Check sheet for the drawn part. Datum: minimum x, y, z corner. Units: mm. Round coordinates to 2 decimals unless told otherwise and drop trailing zeros. Write each loop counter-clockwise with the first axis right and the second up, starting at its lowest first coordinate (ties: lowest second). Pieces come first, ordered by that corner, then holes. Notation, with made-up numbers: (87, -20.75) - (142, -20.75) arc R22 cw to (142, 13.25) - close; hole circle Ø4 at (-20, 5.5). An arc over 180 degrees is marked (long way). Answer as a JSON object with one key per item and string values.
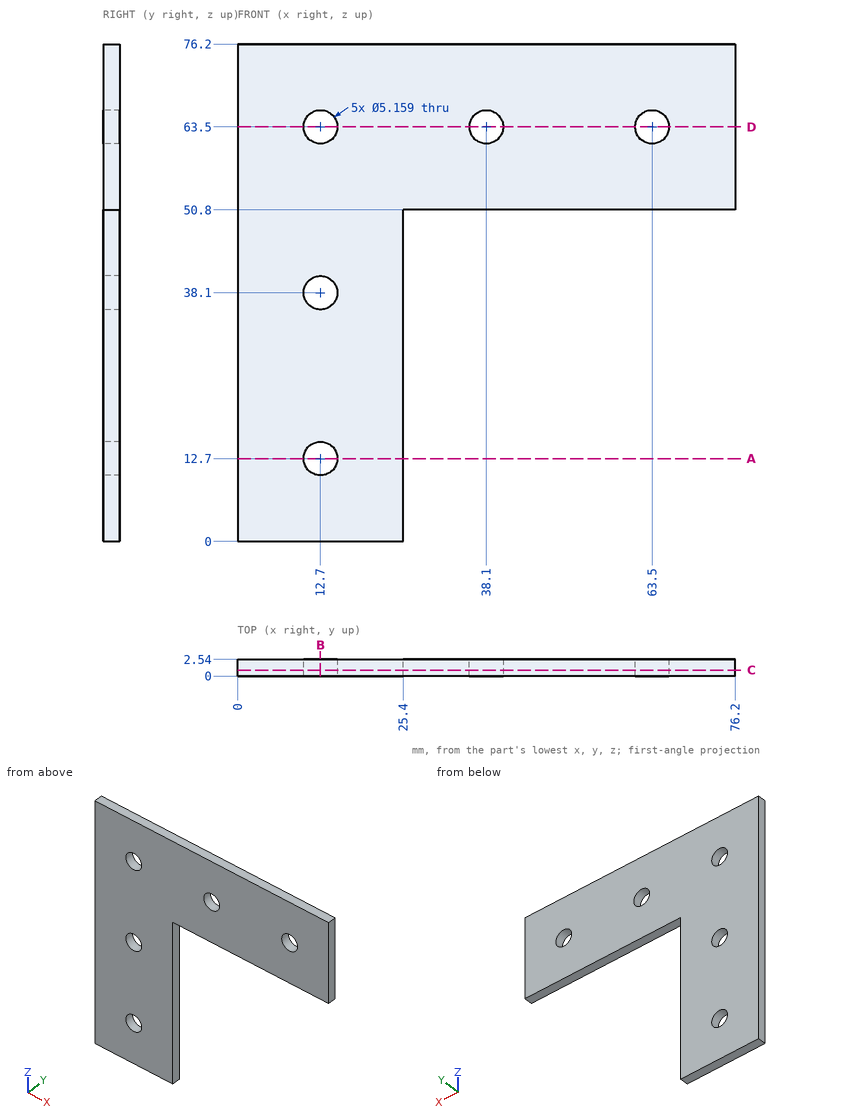
1. Cross-section at D-D (z = 63.5). Record the boundary of the cut face in (x, y).
Completed:
{"outline": "(0, 0) - (10.12, 0) - (10.12, 2.54) - (0, 2.54) - close; (15.28, 0) - (35.52, 0) - (35.52, 2.54) - (15.28, 2.54) - close; (40.68, 0) - (60.92, 0) - (60.92, 2.54) - (40.68, 2.54) - close; (66.08, 0) - (76.2, 0) - (76.2, 2.54) - (66.08, 2.54) - close"}
2. Cross-section at C-C (y = 0.9). Record the boundary of the cut face in (x, z), plus the area to 3 significant figures.
Completed:
{"outline": "(0, 0) - (25.4, 0) - (25.4, 50.8) - (76.2, 50.8) - (76.2, 76.2) - (0, 76.2) - close; hole circle Ø5.16 at (12.7, 12.7); hole circle Ø5.16 at (12.7, 38.1); hole circle Ø5.16 at (12.7, 63.5); hole circle Ø5.16 at (38.1, 63.5); hole circle Ø5.16 at (63.5, 63.5)", "area": "3,120 mm^2"}
3. Cross-section at B-B (x = 12.7). Record the boundary of the cut face in (y, z), plus the area to 3 significant figures.
Completed:
{"outline": "(0, 0) - (2.54, 0) - (2.54, 10.12) - (0, 10.12) - close; (0, 15.28) - (2.54, 15.28) - (2.54, 35.52) - (0, 35.52) - close; (0, 40.68) - (2.54, 40.68) - (2.54, 60.92) - (0, 60.92) - close; (0, 66.08) - (2.54, 66.08) - (2.54, 76.2) - (0, 76.2) - close", "area": "154 mm^2"}
4. Material ranges on probe 1 along Z at (x, y) = (12.7, 1); probe 2 along Z at (x, y) = (11, 1.55); probe 3 along X at (y, z) = (1.35, 62.5), recorded low to high. Write a range as from..to.
Completed:
{"probe 1": "z = 0..10.12, 15.28..35.52, 40.68..60.92, 66.08..76.2", "probe 2": "z = 0..10.76, 14.64..36.16, 40.04..61.56, 65.44..76.2", "probe 3": "x = 0..10.32, 15.08..35.72, 40.48..61.12, 65.88..76.2"}
5. Go/stop test with flat-tipped pins: pin 1 (8.5 mm diameter, centred on x = 38.1, z = 63.5, fed in from -Y); pin 2 (1 mm diameter, centred on y = 1, z = 27.5, fed in from +X); pin 3 (1 mm diameter, centred on x = 63, y = 0.5, fed in from -Z). Record where each tip stops, or that it passes through.
Completed:
{"pin 1": "stops at y = 0", "pin 2": "stops at x = 25.4", "pin 3": "stops at z = 50.8"}
6. Cross-section at A-A (z = 12.7). Record the boundary of the cut face in (x, y).
Completed:
{"outline": "(0, 0) - (10.12, 0) - (10.12, 2.54) - (0, 2.54) - close; (15.28, 0) - (25.4, 0) - (25.4, 2.54) - (15.28, 2.54) - close"}
